Verification items for the finished model (mm, model axes). Round coordinates to 2 decimals unless told otherwise and drop trailing zeros. Write each loop counter-clockwise with the first axis right and the second up, starting at its lowest first coordinate (ties: lowest second). Pieces come first, ordered by that corner, then holes. Notation, with made-up numbers: M -38,-33 L -20,-33 A33 ccw -20,5 Z; hole C 13.25,47 d9. An arc over 180 degrees is marked long. One line per question, with ' | ' between items.
from build123d import *

# Parameters (mm, degrees)
SKETCH1_W           = 450
SKETCH1_H           = 300
BOSS_EXTRUDE1_DEPTH = 9
CUT_EXTRUDE2_DEPTH  = 1
SKETCH5_R           = 4
BOSS_EXTRUDE3_DEPTH = 90


with BuildPart() as part:
    # Sketch1 → Boss-Extrude1 (new, symmetric)
    with BuildSketch(Plane.XY):
        Rectangle(SKETCH1_W, SKETCH1_H)
    extrude(amount=BOSS_EXTRUDE1_DEPTH, both=True)

    # Sketch3 → Cut-Extrude2 (cut)
    with BuildSketch(Plane.XY.offset(9)):
        Polygon((-225, 1), (-225, -1), (-76, -1), (-76, -150), (-74, -150), (-74, -1), (74, -1), (74, -150), (76, -150), (76, -1), (225, -1), (225, 1), (76, 1), (76, 150), (74, 150), (74, 1), (-74, 1), (-74, 150), (-76, 150), (-76, 1), align=None)
    cut_extrude2 = extrude(amount=-CUT_EXTRUDE2_DEPTH, mode=Mode.SUBTRACT)

    # Sketch5 → Boss-Extrude3 (add)
    with BuildSketch(Plane.XY.offset(9)):
        with Locations((-133, 128)):
            Circle(SKETCH5_R)
        with Locations((17, 128)):
            Circle(SKETCH5_R)
        with Locations((167, 128)):
            Circle(SKETCH5_R)
        with Locations((17, -22)):
            Circle(SKETCH5_R)
        with Locations((167, -22)):
            Circle(SKETCH5_R)
        with Locations((-133, -22)):
            Circle(SKETCH5_R)
    boss_extrude3 = extrude(amount=BOSS_EXTRUDE3_DEPTH)

    # Mirror1: Cut-Extrude2, Boss-Extrude3 across plane
    add(cut_extrude2.mirror(Plane.XY), mode=Mode.SUBTRACT)
    add(boss_extrude3.mirror(Plane.XY))


solid = part.part
1. Section check C-C, the plane x = 82. Record the cut outline in (y, z).
Results:
outline: M -150,-9 L -1,-9 L -1,-8 L 1,-8 L 1,-9 L 150,-9 L 150,9 L 1,9 L 1,8 L -1,8 L -1,9 L -150,9 Z
2. Section check B-B, the plane y = -31. Record the cut outline in (x, z).
Results:
outline: M -225,-9 L -76,-9 L -76,-8 L -74,-8 L -74,-9 L 74,-9 L 74,-8 L 76,-8 L 76,-9 L 225,-9 L 225,9 L 76,9 L 76,8 L 74,8 L 74,9 L -74,9 L -74,8 L -76,8 L -76,9 L -225,9 Z
3. Go/stop test with flat-tipped pins: P1, Ø1.5, axis at x = -174, y = 86.5, coming from the +Z side; P2, Ø12, axis at x = -142, y = 20, coming from the -Z side. Record where each tip stops, or that it passes through.
Results:
P1: stops at z = 9 | P2: stops at z = -9
4. Thickness scan on line 1 (Z direction, x = -169, y = -89.5). Record the ranges inside material, lowest first.
Results:
line 1: z = -9 to 9
5. Section check A-A, the plane z = 20.5. Record the cut outline in (x, y), then the cut area to 3 significant figures.
Results:
outline: C -133,-22 d8; C -133,128 d8; C 17,-22 d8; C 17,128 d8; C 167,-22 d8; C 167,128 d8 | area: 302 mm2
6. Mould release check, pull along Y, two halves, no side actions. Record for faces 1 (the face through (-225, -2, 0)), 2 (the face through (-1.1, 0.7, 8)), 3 (the face through (-3, -150, 0)): pulls with the +Y half, pulls with the -Y half, needs draft (parallel to the pull), parting line crosses it, or undercut.
Results:
face 1: needs draft | face 2: undercut | face 3: pulls with the -Y half
